```python
from build123d import *

# Parameters (mm, degrees)
SKETCH1_W               = 141.5
SKETCH1_H               = 20
BOSS_EXTRUDE1_DEPTH     = 2
SKETCH2_W               = 2
SKETCH2_H               = 20
BOSS_EXTRUDE2_DEPTH     = 11
SKETCH3_W               = 20
SKETCH3_H               = 1.5
BOSS_EXTRUDE3_DEPTH     = 1.5
CHAMFER1_SIZE           = 1
SKETCH4_W               = 20
SKETCH4_H               = 1.5
BOSS_EXTRUDE4_DEPTH     = 1.5
CHAMFER2_SIZE           = 1
CUT_EXTRUDE1_DEPTH      = 1.5
CUT_EXTRUDE1_DEPTH_BACK = 11.5
SKETCH5_W               = 12
SKETCH5_H               = 14.324896111
SKETCH6_W               = 2.5
SKETCH6_H               = 10
BOSS_EXTRUDE5_DEPTH     = 22
SKETCH7_W               = 2.8
SKETCH7_H               = 10
BOSS_EXTRUDE6_DEPTH     = 3
SKETCH8_W               = 2.8
SKETCH8_H               = 10
BOSS_EXTRUDE7_DEPTH     = 3
CHAMFER3_SIZE           = 1
SKETCH9_W               = 2
SKETCH9_H               = 17
BOSS_EXTRUDE8_DEPTH     = 1
FILLET1_R               = 1
FILLET2_R               = 2
SKETCH11_W              = 119.5
SKETCH11_H              = 10
CUT_EXTRUDE2_DEPTH      = 10
FILLET3_R               = 3


with BuildPart() as part:
    # Sketch1 → Boss-Extrude1 (new body)
    with BuildSketch(Plane(origin=(0, 0, 0), x_dir=(1, 0, 0), z_dir=(0, 1, 0))):
        Rectangle(SKETCH1_W, SKETCH1_H)
    extrude(amount=BOSS_EXTRUDE1_DEPTH)

    # Sketch2 → Boss-Extrude2 (add)
    with BuildSketch(Plane(origin=(0, 2, 0), x_dir=(1, 0, 0), z_dir=(0, 1, 0))):
        with Locations((69.75, 0)):
            Rectangle(SKETCH2_W, SKETCH2_H)
        with Locations((-69.75, 0)):
            Rectangle(SKETCH2_W, SKETCH2_H)
    extrude(amount=BOSS_EXTRUDE2_DEPTH)

    # Sketch3 → Boss-Extrude3 (add)
    with BuildSketch(Plane.ZY.offset(-68.75)):
        with Locations((0, 12.25)):
            Rectangle(SKETCH3_W, SKETCH3_H)
    extrude(amount=BOSS_EXTRUDE3_DEPTH)

    # Chamfer1
    chamfer1_edges = [part.edges().sort_by_distance(p)[0] for p in [
        (67.25, 13, 0),
    ]]
    chamfer(chamfer1_edges, length=CHAMFER1_SIZE)

    # Sketch4 → Boss-Extrude4 (add)
    with BuildSketch(Plane(origin=(-68.75, 0, 0), x_dir=(0, 0, -1), z_dir=(1, 0, 0))):
        with Locations((0, 12.25)):
            Rectangle(SKETCH4_W, SKETCH4_H)
    extrude(amount=BOSS_EXTRUDE4_DEPTH)

    # Chamfer2
    chamfer2_edges = [part.edges().sort_by_distance(p)[0] for p in [
        (-67.25, 13, 0),
    ]]
    chamfer(chamfer2_edges, length=CHAMFER2_SIZE)

    # Sketch5 → Cut-Extrude1 (cut, two sides: drawn at the far end of the back side and taken through both)
    with BuildSketch(Plane(origin=(-68.75, 0, 0), x_dir=(0, 0, -1), z_dir=(1, 0, 0)).offset(-CUT_EXTRUDE1_DEPTH_BACK)):
        with Locations((0, 12.162448056)):
            Rectangle(SKETCH5_W, SKETCH5_H)
    extrude(amount=CUT_EXTRUDE1_DEPTH + CUT_EXTRUDE1_DEPTH_BACK, mode=Mode.SUBTRACT)

    # Sketch6 → Boss-Extrude5 (add)
    with BuildSketch(Plane.ZY.offset(70.75)):
        with Locations((-7.25, 8)):
            Rectangle(SKETCH6_W, SKETCH6_H)
        with Locations((7.25, 8)):
            Rectangle(SKETCH6_W, SKETCH6_H)
    extrude(amount=BOSS_EXTRUDE5_DEPTH)

    # Sketch7 → Boss-Extrude6 (add)
    with BuildSketch(Plane(origin=(0, 0, 6), x_dir=(-1, 0, 0), z_dir=(0, 0, -1))):
        with Locations((91.35, 8)):
            Rectangle(SKETCH7_W, SKETCH7_H)
    extrude(amount=BOSS_EXTRUDE6_DEPTH)

    # Sketch8 → Boss-Extrude7 (add)
    with BuildSketch(Plane.XY.offset(-6)):
        with Locations((-91.35, 8)):
            Rectangle(SKETCH8_W, SKETCH8_H)
    extrude(amount=BOSS_EXTRUDE7_DEPTH)

    # Chamfer3
    chamfer3_edges = [part.edges().sort_by_distance(p)[0] for p in [
        (-92.75, 8, 3),
        (-92.75, 8, -3),
    ]]
    chamfer(chamfer3_edges, length=CHAMFER3_SIZE)

    # Sketch9 → Boss-Extrude8 (add)
    with BuildSketch(Plane.XZ.offset(-3)):
        with Locations((-79.75, 0)):
            Rectangle(SKETCH9_W, SKETCH9_H)
    extrude(amount=-BOSS_EXTRUDE8_DEPTH)

    # Fillet1
    fillet1_edges = [part.edges().sort_by_distance(p)[0] for p in [
        (-80.75, 3.5, -6),
        (-80.75, 3.5, 6),
        (-78.75, 3.5, -6),
        (-78.75, 3.5, 6),
    ]]
    fillet(fillet1_edges, radius=FILLET1_R)

    # Fillet2
    fillet2_edges = [part.edges().sort_by_distance(p)[0] for p in [
        (68.75, 2, 0),
        (-68.75, 2, 0),
    ]]
    fillet(fillet2_edges, radius=FILLET2_R)

    # Sketch11 → Cut-Extrude2 (cut)
    with BuildSketch(Plane(origin=(0, 2, 0), x_dir=(1, 0, 0), z_dir=(0, 1, 0))):
        Rectangle(SKETCH11_W, SKETCH11_H)
    extrude(amount=-CUT_EXTRUDE2_DEPTH, mode=Mode.SUBTRACT)

    # Fillet3
    fillet3_edges = [part.edges().sort_by_distance(p)[0] for p in [
        (-59.75, 1, 5),
        (-59.75, 1, -5),
        (59.75, 1, -5),
        (59.75, 1, 5),
    ]]
    fillet(fillet3_edges, radius=FILLET3_R)


solid = part.part
```
Read the model definition and answer for the solid it produces. Units are mm, in the model's axes. A direction names the side the tool comes from. Round coordinates to 2 decimals unless told otherwise and drop trailing zeros. Write each loop counter-clockwise with the first axis right and the second up, starting at its lowest first coordinate (ties: lowest second). Pieces come first, ordered by that corner, then holes. Notation, with made-up numbers: (-3.5, 77) -> (21.5, 77) arc R28 ccw to (21.5, 110) -> close; hole circle Ø11 at (50.5, -3.5). An arc over 180 degrees is marked (long way). Answer in a Markdown table with one row per item. Add a question column.
1) Find section A-A, the plane y = 6.5. Determine the outline of the cut face in (x, z).
2) Consider line 1 (Z direction, x = -76, y = 10.25); line 2 (X direction, y = 9, z = 4.25); line 3 (X direction, y = 4.5, z = 1.75). Determine where each line is inside the solid, lowest interval first.
3) Find section B-B, the plane x = -74.5. Determine the outline of the cut face in (y, z), and give its area (3 significant figures).
4) Determine the mould class of faces 6 (the face through (-92.75, 8, 6)), 7 (the face through (-78, 8, -6)), 8 (the face through (-80, 13, 7)) for opening direction X: pulls with the +X half, pulls with the -X half, needs draft (parallel to the pull), parting line crosses it, or undercut.
5) Find section D-D, the plane x = 32.5. Determine the outline of the cut face in (y, z), and give its area (3 significant figures).
6) Given P1, Ø2, axis at x = -91, y = 9.5, coming from the -Z side; P2, Ø1, axis at x = -19, y = 3, coming from the +Z side; P3, Ø1, axis at y = 2, z = 0, coming from the -X side; P4, Ø6, axis at x = -19, z = 5.5, coming from the +Y side, each flat-ended and moving along its own axis, determine where each tip first touches the part or whether it passes through.
7) Find section C-C, the plane z = -0.5. Determine the outline of the cut face in (x, y), and give its area (3 significant figures).
8) Which of the six approach directions +Z, -Z, +X, -X, +Y, -Y give full straight-line access (tool end or side, diameter ignored) to faces 1 (the face through (-68.75, 4.4, 0.1)), 2 (the face through (-80, 4, 0)), 3 (the face through (58.85, 0.99, 4.14)), 4 (the face through (-82, 8, -8.5)), 5 (the face through (-1, 2, -7))?
Findings below:
| question | item | result |
|---|---|---|
| 1 | outline | (-92.75, -8.5) -> (-70.75, -8.5) -> (-70.75, -10) -> (-68.75, -10) -> (-68.75, -6) -> (-89.95, -6) -> (-89.95, -3) -> (-91.75, -3) -> (-92.75, -4) -> close; (-92.75, 4) -> (-91.75, 3) -> (-89.95, 3) -> (-89.95, 6) -> (-68.75, 6) -> (-68.75, 10) -> (-70.75, 10) -> (-70.75, 8.5) -> (-92.75, 8.5) -> close; (68.75, -10) -> (70.75, -10) -> (70.75, 10) -> (68.75, 10) -> close |
| 2 | line 1 | -8.5 to -6, 6 to 8.5 |
| 2 | line 2 | -92.75 to -89.95, 68.75 to 70.75 |
| 2 | line 3 | -70.75 to -68.75, 68.75 to 70.75 |
| 3 | outline | (3, -8.5) -> (13, -8.5) -> (13, -6) -> (3, -6) -> close; (3, 6) -> (13, 6) -> (13, 8.5) -> (3, 8.5) -> close |
| 3 | area | 50.0 mm² |
| 4 | face 6 | pulls with the -X half |
| 4 | face 7 | undercut |
| 4 | face 8 | needs draft |
| 5 | outline | (0, -10) -> (2, -10) -> (2, -5) -> (0, -5) -> close; (0, 5) -> (2, 5) -> (2, 10) -> (0, 10) -> close |
| 5 | area | 20.0 mm² |
| 6 | P1 | z = -8.5 |
| 6 | P2 | through |
| 6 | P3 | x = -70.75 |
| 6 | P4 | y = 2 |
| 7 | outline | (-80.75, 3) -> (-78.75, 3) -> (-78.75, 4) -> (-80.75, 4) -> close; (-70.75, 0) -> (-59.75, 0) -> (-59.75, 2) -> (-66.75, 2) arc R2 cw to (-68.75, 4) -> (-68.75, 5) -> (-70.75, 5) -> close; (59.75, 0) -> (70.75, 0) -> (70.75, 13) -> (68.25, 13) -> (67.25, 12) -> (67.25, 11.5) -> (68.75, 11.5) -> (68.75, 4) arc R2 cw to (66.75, 2) -> (59.75, 2) -> close |
| 7 | area | 77.5 mm² |
| 8 | face 1 | +Z, -Z |
| 8 | face 2 | +Y |
| 8 | face 3 | +Y, -Y |
| 8 | face 4 | -Z, -X, +Y, -Y |
| 8 | face 5 | +Z, -Z, +Y |
